Build history of the part. All positions in model axes, mm. Give positions to 0.01 mm unless a question says otherwise; leave off trailing zeros. Order: outer loops, then holes, each group sorted by start corner. A loop starts at its lowest first (then second) coordinate and runs counter-clockwise, first axis right, second up. Notation, with made-up numbers: (64.25, -5.75) - (82.25, -5.75) arc R14 cw to (82.25, 6.25) - close; hole circle Ø6 at (14, 64). An arc over 180 degrees is marked (long way). Use a Markdown table: item, result. Add a question column.
(1) Slice it at C-C (y = 95.5). Write the cut outline in (x, z).
(2) Slice it at B-B (z = 43.5). Write the cut outline in (x, y).
(3) Flat gauge pins, fed straight in: pin 1 (6 mm diameter, centred on x = 5, y = 156, fed in from -Z); pin 2 (4 mm diameter, centred on x = 7.5, y = 389, fed in from +Z); pin 3 (1.5 mm diameter, centred on y = 451.5, z = 138, fed in from -X); pin 4 (6.5 mm diameter, centred on x = 6.5, z = 146, fed in from +Y). Where does each tip first touch, or does it go through?
(4) Slice it at A-A (y = 220). Write the cut outline in (x, z), then the cut area to 3 significant figures.
(5) Wall check: line 1 (Z direction, x = 7, y = 158); line 2 (Z direction, x = 7.5, y = 229); line 3 (Z direction, x = 7.75, y = 133.5). Give the ranges that are in metal, low to high.
(6) Slice it at D-D (x = 8.25). Count the separate pieces of the cut face and the enclosed holes in it, then the cut area to 3 significant figures.
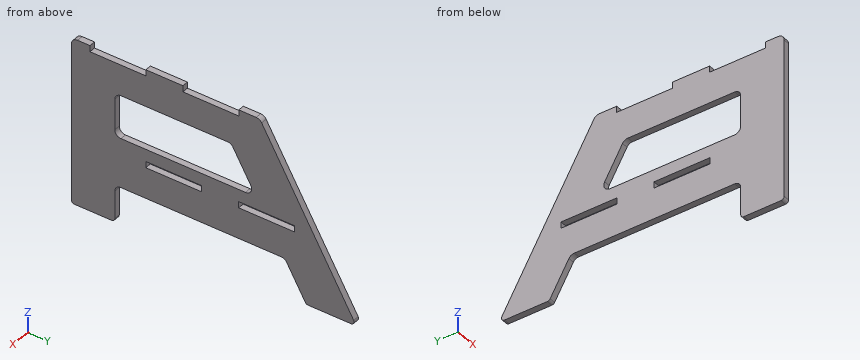
from build123d import *

# Parameters (mm, degrees)
F0_W     = 114.554
F0_H     = 12.954
F1_DEPTH = 12.7


with BuildPart() as f1:
    # F0 (on Right) → F1 (new body)
    with BuildSketch(Plane.YZ):
        with BuildLine():
            ThreePointArc((0, 6.35), (1.859872, 1.859872), (6.35, 0))
            Line((6.35, 0), (82.55, 0))
            ThreePointArc((82.55, 0), (87.040128, 1.859872), (88.9, 6.35))
            Line((88.9, 6.35), (88.9, 63.5))
            ThreePointArc((88.9, 63.5), (92.619744, 72.480256), (101.6, 76.2))
            Line((101.6, 76.2), (430.220683, 76.2))
            ThreePointArc((430.220683, 76.2), (436.570683, 74.498523), (441.219206, 69.85))
            Line((441.219206, 69.85), (479.714035, 3.175))
            ThreePointArc((479.714035, 3.175), (482.038296, 0.850739), (485.213296, 0))
            Line((485.213296, 0), (573.201477, 0))
            ThreePointArc((573.201477, 0), (578.700739, 3.175), (578.700739, 9.525))
            Line((578.700739, 9.525), (389.892767, 336.55))
            ThreePointArc((389.892767, 336.55), (385.244244, 341.198523), (378.894244, 342.9))
            Line((378.894244, 342.9), (343.154, 342.9))
            Line((343.154, 342.9), (343.154, 330.2))
            Line((343.154, 330.2), (228.6, 330.2))
            Line((228.6, 330.2), (228.6, 342.9))
            Line((228.6, 342.9), (152.654, 342.9))
            Line((152.654, 342.9), (152.654, 330.2))
            Line((152.654, 330.2), (38.1, 330.2))
            Line((38.1, 330.2), (38.1, 342.9))
            Line((38.1, 342.9), (12.7, 342.9))
            ThreePointArc((12.7, 342.9), (3.719744, 339.180256), (0, 330.2))
            Line((0, 330.2), (0, 6.35))
        make_face()
        with Locations((209.677, 146.177)):
            Rectangle(F0_W, F0_H, mode=Mode.SUBTRACT)
        with Locations((400.177, 146.177)):
            Rectangle(F0_W, F0_H, mode=Mode.SUBTRACT)
        with BuildLine():
            Line((88.9, 190.5), (88.9, 254))
            ThreePointArc((88.9, 254), (92.619744, 262.980256), (101.6, 266.7))
            Line((101.6, 266.7), (320.235457, 266.7))
            ThreePointArc((320.235457, 266.7), (326.585457, 264.998523), (331.23398, 260.35))
            Line((331.23398, 260.35), (367.895722, 196.85))
            ThreePointArc((367.895722, 196.85), (367.895722, 184.15), (356.897199, 177.8))
            Line((356.897199, 177.8), (101.6, 177.8))
            ThreePointArc((101.6, 177.8), (92.619744, 181.519744), (88.9, 190.5))
        make_face(mode=Mode.SUBTRACT)
    extrude(amount=F1_DEPTH)


solid = f1.part
Solution:
| question | item | result |
|---|---|---|
| 1 | outline | (0, 74.64) - (12.7, 74.64) - (12.7, 179.36) - (0, 179.36) - close; (0, 265.14) - (12.7, 265.14) - (12.7, 330.2) - (0, 330.2) - close |
| 2 | outline | (0, 0) - (12.7, 0) - (12.7, 88.9) - (0, 88.9) - close; (0, 456.43) - (12.7, 456.43) - (12.7, 559.09) - (0, 559.09) - close |
| 3 | pin 1 | z = 76.2 |
| 3 | pin 2 | z = 339.98 |
| 3 | pin 3 | x = 0 |
| 3 | pin 4 | y = 501.78 |
| 4 | outline | (0, 76.2) - (12.7, 76.2) - (12.7, 139.7) - (0, 139.7) - close; (0, 152.65) - (12.7, 152.65) - (12.7, 177.8) - (0, 177.8) - close; (0, 266.7) - (12.7, 266.7) - (12.7, 342.9) - (0, 342.9) - close |
| 4 | area | 2,090 mm2 |
| 5 | line 1 | 76.2 to 139.7, 152.65 to 177.8, 266.7 to 342.9 |
| 5 | line 2 | 76.2 to 139.7, 152.65 to 177.8, 266.7 to 330.2 |
| 5 | line 3 | 76.2 to 177.8, 266.7 to 330.2 |
| 6 | separate pieces | 1 |
| 6 | enclosed holes | 3 |
| 6 | area | 109,000 mm2 |
